from build123d import *

# Parameters (mm, degrees)
SKETCH_1_R      = 8
EXTRUDE_1_DEPTH = 2


with BuildPart() as part:
    # 草圖1 → 填料-伸長1 (new body)
    with BuildSketch(Plane(origin=(0, 0, 0), x_dir=(1, 0, 0), z_dir=(0, 1, 0))):
        Polygon((12.5, 20.511459459), (25, 20.511459459), (25, -20.511459459), (-25, -20.511459459), (-25, 20.511459459), (-12.5, 20.511459459), (-12.5, 22.511459459), (12.5, 22.511459459), align=None)
        with Locations((-13.48, 0)):
            Circle(SKETCH_1_R, mode=Mode.SUBTRACT)
        with Locations((13.48, 0)):
            Circle(SKETCH_1_R, mode=Mode.SUBTRACT)
    extrude(amount=EXTRUDE_1_DEPTH)


solid = part.part
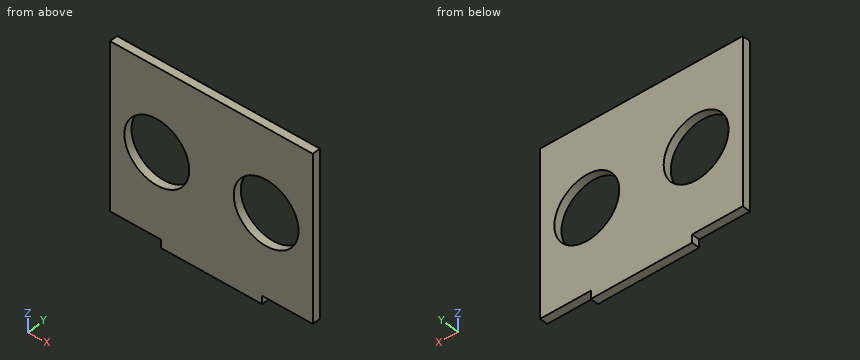
Source: CAD feature listing. Evaluate the final solid. Frame: model axes, mm. Give positions to 0.01 mm unless a question says otherwise; leave off trailing zeros. Write each loop counter-clockwise with the first axis right and the second up, starting at its lowest first coordinate (ties: lowest second). Pieces come first, ordered by that corner, then holes. Notation, with made-up numbers: (-14, 55) -> (22, 55) arc R20 ccw to (22, 89) -> close; hole circle Ø1 at (37, 1.5). An arc over 180 degrees is marked (long way). Return JSON: item names as keys, results as strings. Group by question number.
1. Pin query (flat end, axial travel): pin 1 Ø9.5 at (x, z) = (-13.48, 0) entering from -Y; pin 2 Ø1 at (x, y) = (-18.5, 0.5) entering from -Z. Return the tip coordinate at first contact, or that it passes through.
2. Section D-D, the plane x = 6.5. Output: boundary loops of the cut face in (y, z), then the cut area to 3 significant figures.
3. Section B-B, the plane y = 0.7. Output: boundary loops of the cut face in (x, z), then the cut area to 3 significant figures.
4. Section A-A, the plane z = 0. Output: boundary loops of the cut face in (x, y), then the cut area to 3 significant figures.
5. Material intervals for line 1 (X direction, y = 0.4, z = 0); line 2 (Z direction, x = 13.48, y = 1.2); line 3 (X direction, y = 1.75, z = 4), sorted ascending. Write a range as from..to.
6. Section C-C, the plane x = -13.48. Output: boundary loops of the cut face in (y, z), then the cut area to 3 significant figures.
Determined:
{
 "1": {"pin 1": "passes through", "pin 2": "stops at z = -20.51"},
 "2": {"outline": "(0, -22.51) -> (2, -22.51) -> (2, -3.91) -> (0, -3.91) -> close; (0, 3.91) -> (2, 3.91) -> (2, 20.51) -> (0, 20.51) -> close", "area": "70.4 mm2"},
 "3": {"outline": "(-25, -20.51) -> (-12.5, -20.51) -> (-12.5, -22.51) -> (12.5, -22.51) -> (12.5, -20.51) -> (25, -20.51) -> (25, 20.51) -> (-25, 20.51) -> close; hole circle Ø16 at (-13.48, 0); hole circle Ø16 at (13.48, 0)", "area": "1,700 mm2"},
 "4": {"outline": "(-25, 0) -> (-21.48, 0) -> (-21.48, 2) -> (-25, 2) -> close; (-5.48, 0) -> (5.48, 0) -> (5.48, 2) -> (-5.48, 2) -> close; (21.48, 0) -> (25, 0) -> (25, 2) -> (21.48, 2) -> close", "area": "36.0 mm2"},
 "5": {"line 1": "x = -25..-21.48, -5.48..5.48, 21.48..25", "line 2": "z = -20.51..-8, 8..20.51", "line 3": "x = -25..-20.41, -6.55..6.55, 20.41..25"},
 "6": {"outline": "(0, -20.51) -> (2, -20.51) -> (2, -8) -> (0, -8) -> close; (0, 8) -> (2, 8) -> (2, 20.51) -> (0, 20.51) -> close", "area": "50.0 mm2"}
}
